```python
from build123d import *

# Parameters (mm, degrees)
F0_R     = 19.05
F0_R_2   = 17.78
F1_DEPTH = 52.07
F2_R     = 0.635
F3_R     = 10.16
F3_R_2   = 7.62
F4_DEPTH = 30.48
F5_R     = 7.62
F6_DEPTH = 30.481
F8_DEPTH = 25.4


with BuildPart() as f1:
    # F0 (on Right) → F1 (new body, symmetric)
    with BuildSketch(Plane.YZ):
        Circle(F0_R)
        Circle(F0_R_2, mode=Mode.SUBTRACT)
    extrude(amount=F1_DEPTH, both=True)

    # F2
    f2_edges = [f1.edges().sort_by_distance(p)[0] for p in [
        (52.07, -19.05, 0),
        (-52.07, -19.05, 0),
    ]]
    fillet(f2_edges, radius=F2_R)

    # F3 (on Top) → F4 (join)
    with BuildSketch(Plane.XY):
        Circle(F3_R)
        Circle(F3_R_2, mode=Mode.SUBTRACT)
    extrude(amount=F4_DEPTH)

    # F5 (on Top) → F6 (cut, through all)
    with BuildSketch(Plane.XY):
        Circle(F5_R)
    extrude(amount=F6_DEPTH, mode=Mode.SUBTRACT)

    # F7 (on Right) → F8 (cut, symmetric)
    with BuildSketch(Plane.YZ):
        with BuildLine():
            Line((-10.16, 12.7), (-10.16, 14.591189))
            ThreePointArc((-10.16, 14.591189), (0, -17.78), (10.16, 14.591189))
            Line((10.16, 14.591189), (10.16, 12.7))
            Line((10.16, 12.7), (-10.16, 12.7))
        make_face()
    extrude(amount=F8_DEPTH, both=True, mode=Mode.SUBTRACT)


solid = f1.part
```
Geometry check sheet. Reference: the model listing, model coordinates, mm. A direction names the side the tool comes from. Give positions to 0.01 mm unless a question says otherwise; leave off trailing zeros. Order: outer loops, then holes, each group sorted by start corner. A loop starts at its lowest first (then second) coordinate and runs counter-clockwise, first axis right, second up. Notation, with made-up numbers: (87, -32.5) -> (138, -32.5) arc R28 cw to (138, 5.5) -> close; hole circle Ø8 at (-14, 83). An arc over 180 degrees is marked (long way). Write each question's results on one line, items separated by ' | '. Start each with the question number.
(1) Sectioned sample at A-A (z = 0). Enter the section's corners in (x, y) (3 decimals).
(2) Sectioned sample at B-B (y = 0). Enter the section's corners in (x, z) (3 decimals).
(3) Sectioned sample at C-C (x = -44). Enter the section's corners in (y, z), plus the area to 3 significant figures.
(4) Mould release check, pull along Z, two halves, no side actions. Record for faces 1 (the face through (0.72, -4.13, -18.597)), 2 (the face through (-52.07, -10, 15)), 3 (the face through (8, -1, 12.7)): pulls with the +Z half, pulls with the -Z half, needs draft (parallel to the pull), parting line crosses it, or undercut.
(5) Access from +Z, -Z, +X, -X, +Y, -Y to the whole of each face (thin tool, end or side, straight path). Record for faces 4 (the face through (-7.488, 6.867, 14.641)), 5 (the face through (-8.063, -6.182, 23.197)), 6 (the face through (1, 8, 30.48)).
(6) Sectioned sample at D-D (x = 0). Enter the section's corners in (y, z), plus the area to 3 significant figures.
(7) Scan lines: line 1 (Y direction, x = 0, z = 18); line 2 (Z direction, x = 48.5, y = 0.5). Record each from-to range of solid material in increasing order.
(8) Gauge pin test, flat ends, axial feed: P1, Ø2, axis at x = 25.5, z = 3, coming from the +Y side; P2, Ø2, axis at x = 33, y = 12.5, coming from the +Z side; P3, Ø8, axis at x = -10.5, z = 7, coming from the +Y side. Record the tip position at first contact, or that the pin passes through.
Answer below:
1) outline: (-52.07, -18.415) arc R0.635 ccw to (-51.435, -19.05) -> (51.435, -19.05) arc R0.635 ccw to (52.07, -18.415) -> (52.07, -17.78) -> (-52.07, -17.78) -> close; (-52.07, 17.78) -> (52.07, 17.78) -> (52.07, 18.415) arc R0.635 ccw to (51.435, 19.05) -> (-51.435, 19.05) arc R0.635 ccw to (-52.07, 18.415) -> close
2) outline: (-52.07, -18.415) arc R0.635 ccw to (-51.435, -19.05) -> (51.435, -19.05) arc R0.635 ccw to (52.07, -18.415) -> (52.07, -17.78) -> (-52.07, -17.78) -> close; (-52.07, 17.78) -> (-10.16, 17.78) -> (-10.16, 12.7) -> (-7.62, 12.7) -> (-7.62, 30.48) -> (-10.16, 30.48) -> (-10.16, 19.05) -> (-51.435, 19.05) arc R0.635 ccw to (-52.07, 18.415) -> close; (7.62, 12.7) -> (10.16, 12.7) -> (10.16, 17.78) -> (52.07, 17.78) -> (52.07, 18.415) arc R0.635 ccw to (51.435, 19.05) -> (10.16, 19.05) -> (10.16, 30.48) -> (7.62, 30.48) -> close
3) outline: circle Ø38.1 at (0, 0); hole circle Ø35.56 at (0, 0) | area: 147 mm2
4) face 1: parting line crosses it | face 2: needs draft | face 3: undercut
5) face 4: none | face 5: +Z | face 6: +Z, +X, -X, +Y, -Y
6) outline: (-10.16, 12.7) -> (-7.62, 12.7) -> (-7.62, 30.48) -> (-10.16, 30.48) -> (-10.16, 16.11) arc R19.05 ccw (long way) to (10.16, 16.11) -> (10.16, 30.48) -> (7.62, 30.48) -> (7.62, 12.7) -> (10.16, 12.7) -> (10.16, 14.59) arc R17.78 cw (long way) to (-10.16, 14.59) -> close | area: 210 mm2
7) line 1: -10.16 to -7.62, 7.62 to 10.16 | line 2: -19.04 to -17.77, 17.77 to 19.04
8) P1: y = 18.94 | P2: z = 15.19 | P3: y = 18.81
